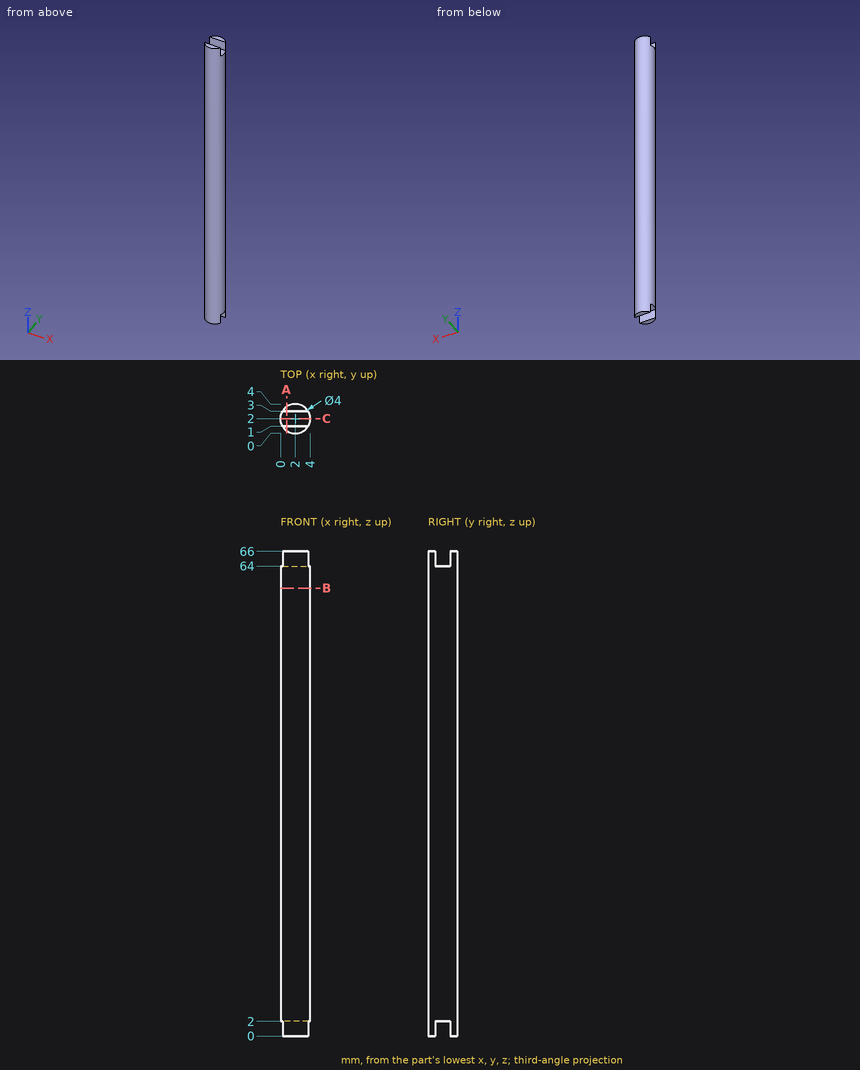
Check sheet for the drawn part. Datum: minimum x, y, z corner. Units: mm. Round coordinates to 2 decimals unless told otherwise and drop trailing zeros. Loops run counter-clockwise (first coordinate to the right, second up) from the corner with the lowest first, then second, coordinate; pieces in that order, holes last.
Item 1: Cross-section at A-A on x = 0.8. Record the boundary of the cut face in (y, z).
Item 2: Thickness scan on line 1 (X direction, y = 2.2, z = 5); line 2 (X direction, y = 3, z = 9); line 3 (Z direction, x = 1, y = 1.4). Record the ranges inside material, lowest first.
Item 3: Cross-section at C-C on y = 2. Record the boundary of the cut face in (x, z).
Item 4: Cross-section at B-B on z = 61. Record the boundary of the cut face in (x, y), then the cut area to 3 significant figures.
Item 5: Gauge pin test, flat ends, axial feed: pin 1 (1.5 mm diameter, centred on y = 1, z = 11.5, fed in from -X); pin 2 (1 mm diameter, centred on x = 1, z = 58.5, fed in from +Y); pin 3 (0.6 mm diameter, centred on x = 2, y = 1.5, fed in from -Z); pin 4 (1 mm diameter, centred on x = 1.5, z = 1.5, fed in from +Y). Record the tip position at first contact, or that the pin passes through.
Answer sheet:
1. outline: (0.4, 0) - (1, 0) - (1, 2) - (3, 2) - (3, 0) - (3.6, 0) - (3.6, 66) - (3, 66) - (3, 64) - (1, 64) - (1, 66) - (0.4, 66) - close
2. line 1: x = 0.01 to 3.99
2. line 2: x = 0.27 to 3.73
2. line 3: z = 2 to 64
3. outline: (0, 2) - (4, 2) - (4, 64) - (0, 64) - close
4. outline: circle Ø4 at (2, 2)
4. area: 12.6 mm2
5. pin 1: stops at x = 0.02
5. pin 2: stops at y = 3.94
5. pin 3: stops at z = 2
5. pin 4: stops at y = 4
